Geometry check sheet. Reference: the model listing, model coordinates, mm. Face numbers are marked on the shaded views. Coordinates: 2 decimals unless noted, no trailing zeros. Write each loop counter-clockwise with the first axis right and the second up, starting at its lowest first coordinate (ties: lowest second). Pieces come first, ordered by that corner, then holes.
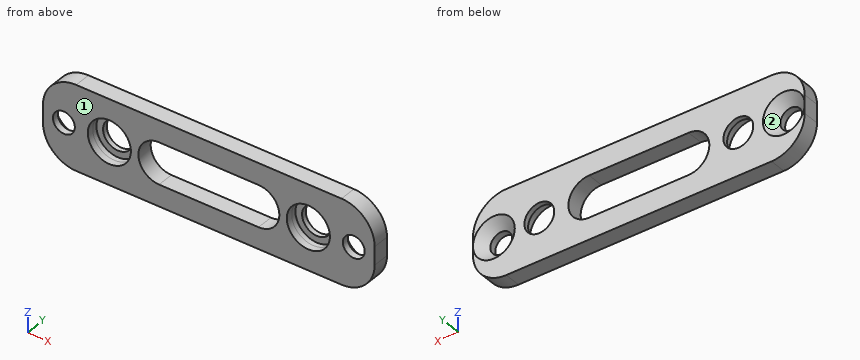
from build123d import *

# Parameters (mm, degrees)
SKETCH1_W                                           = 100
SKETCH1_H                                           = 7
BOSS_EXTRUDE1_DEPTH                                 = 25.5
CSK_FOR_M6_COUNTERSUNK_FLAT_HEAD_SCREW1_D           = 6.6
CSK_FOR_M6_COUNTERSUNK_FLAT_HEAD_SCREW1_CSINK_D     = 12.6
CSK_FOR_M6_COUNTERSUNK_FLAT_HEAD_SCREW1_CSINK_ANGLE = 90
SKETCH2_R                                           = 4.5
CUT_EXTRUDE2_DEPTH                                  = 3
SKETCH2_4_R                                         = 4.5
CUT_EXTRUDE3_DEPTH                                  = 3
SKETCH6_R                                           = 6.5
CUT_EXTRUDE4_DEPTH                                  = 1.5
SKETCH9_R                                           = 6.5
CUT_EXTRUDE5_DEPTH                                  = 5
SKETCH10_W                                          = 100
SKETCH10_H                                          = 25.5
CUT_EXTRUDE6_DEPTH                                  = 2
CUT_EXTRUDE7_DEPTH                                  = 6
FILLET4_R                                           = 10


with BuildPart() as part:
    # Sketch1 → Boss-Extrude1 (new body)
    with BuildSketch(Plane.XY):
        with Locations((50, 3.5)):
            Rectangle(SKETCH1_W, SKETCH1_H)
    extrude(amount=BOSS_EXTRUDE1_DEPTH)

    # CSK for M6 Countersunk Flat Head Screw1 (through all)
    with Locations(Plane(origin=(0, 7, 0), x_dir=(1, 0, 0), z_dir=(0, 1, 0))):
        with Locations((93.7, -12.75), (6.298395044, -12.75)):
            CounterSinkHole(CSK_FOR_M6_COUNTERSUNK_FLAT_HEAD_SCREW1_D / 2, CSK_FOR_M6_COUNTERSUNK_FLAT_HEAD_SCREW1_CSINK_D / 2, counter_sink_angle=CSK_FOR_M6_COUNTERSUNK_FLAT_HEAD_SCREW1_CSINK_ANGLE)

    # Sketch2 → Cut-Extrude2 (cut)
    with BuildSketch(Plane(origin=(0, 7, 0), x_dir=(1, 0, 0), z_dir=(0, 1, 0))):
        with Locations((20, -12.75)):
            Circle(SKETCH2_R)
    extrude(amount=-CUT_EXTRUDE2_DEPTH, mode=Mode.SUBTRACT)

    # Sketch2<4> → Cut-Extrude3 (cut)
    with BuildSketch(Plane(origin=(0, 7, 0), x_dir=(1, 0, 0), z_dir=(0, 1, 0))):
        with Locations((80, -12.75)):
            Circle(SKETCH2_4_R)
        with Locations((20, -12.75)):
            Circle(SKETCH2_4_R)
    extrude(amount=-CUT_EXTRUDE3_DEPTH, mode=Mode.SUBTRACT)

    # Sketch6 → Cut-Extrude4 (cut)
    with BuildSketch(Plane(origin=(0, 4, 0), x_dir=(1, 0, 0), z_dir=(0, 1, 0))):
        with Locations((20, -12.75)):
            Circle(SKETCH6_R)
        with Locations((80, -12.75)):
            Circle(SKETCH6_R)
    extrude(amount=CUT_EXTRUDE4_DEPTH, mode=Mode.SUBTRACT)

    # Sketch9 → Cut-Extrude5 (cut, through all)
    with BuildSketch(Plane(origin=(0, 4, 0), x_dir=(1, 0, 0), z_dir=(0, 1, 0))):
        with Locations((20, -12.75)):
            Circle(SKETCH9_R)
        with Locations((80, -12.75)):
            Circle(SKETCH9_R)
    extrude(amount=-CUT_EXTRUDE5_DEPTH, mode=Mode.SUBTRACT)

    # Sketch10 → Cut-Extrude6 (cut)
    with BuildSketch(Plane.XZ):
        with Locations((50, 12.75)):
            Rectangle(SKETCH10_W, SKETCH10_H)
    extrude(amount=-CUT_EXTRUDE6_DEPTH, mode=Mode.SUBTRACT)

    # Sketch11 → Cut-Extrude7 (cut, through all)
    with BuildSketch(Plane(origin=(0, 7, 0), x_dir=(1, 0, 0), z_dir=(0, 1, 0))):
        with BuildLine():
            Line((35, -19), (65, -19))
            ThreePointArc((65, -19), (71.25, -12.75), (65, -6.5))
            Line((65, -6.5), (35, -6.5))
            ThreePointArc((35, -6.5), (28.75, -12.75), (35, -19))
        make_face()
    extrude(amount=-CUT_EXTRUDE7_DEPTH, mode=Mode.SUBTRACT)

    # Fillet4
    fillet4_edges = [part.edges().sort_by_distance(p)[0] for p in [
        (100, 4.5, 25.5),
        (100, 4.5, 0),
        (0, 4.5, 0),
        (0, 4.5, 25.5),
    ]]
    fillet(fillet4_edges, radius=FILLET4_R)


solid = part.part
1. Sectioned sample at C-C, the plane z = 11. Give the number of separate pieces and of enclosed holes in the cut face, and give its area (3 significant figures).
Computed values:
separate pieces: 6
enclosed holes: 0
area: 102 mm2
2. Sectioned sample at D-D, the plane x = 93.7. Record the boundary of the cut face in (y, z).
Computed values:
outline: (2, 0.71) - (7, 0.71) - (7, 6.45) - (4, 9.45) - (2, 9.45) - close; (2, 16.05) - (4, 16.05) - (7, 19.05) - (7, 24.79) - (2, 24.79) - close
3. Gauge pin test, flat ends, axial feed: pin 1 Ø7 at (x, z) = (20, 12.75) entering from +Y; pin 2 Ø10.5 at (x, z) = (20, 12.75) entering from -Y. Record the tip position at first contact, or that the pin passes through.
Computed values:
pin 1: passes through
pin 2: stops at y = 5.5
4. Sectioned sample at A-A, the plane x = 50.5. Record the boundary of the cut face in (y, z).
Computed values:
outline: (2, 0) - (7, 0) - (7, 6.5) - (2, 6.5) - close; (2, 19) - (7, 19) - (7, 25.5) - (2, 25.5) - close
5. Sectioned sample at B-B, the plane x = 20. Record the boundary of the cut face in (y, z), and give its area (3 significant figures).
Computed values:
outline: (2, 0) - (7, 0) - (7, 8.25) - (5.5, 8.25) - (5.5, 6.25) - (2, 6.25) - close; (2, 19.25) - (5.5, 19.25) - (5.5, 17.25) - (7, 17.25) - (7, 25.5) - (2, 25.5) - close
area: 68.5 mm2
6. Thickness scan on line 1 along X through (y, z) = (3.6, 12.75); line 2 along Z through (x, y) = (42, 4.45); line 3 along Z through (x, y) = (80, 3.2). Record the ranges inside material, lowest first.
Computed values:
line 1: x = 0 to 3, 9.6 to 13.5, 26.5 to 28.75, 71.25 to 73.5, 86.5 to 90.4, 97 to 100
line 2: z = 0 to 6.5, 19 to 25.5
line 3: z = 0 to 6.25, 19.25 to 25.5
7. Draft check along Z on the marked faces 1 and 2. Enter one of: released by +Z, released by -Z, zero draft, split by the parting line, or undercut.
Computed values:
face 1: zero draft
face 2: undercut
